Geometry: final body of the model. Coordinates: model frame, mm. A direction names the side the tool comes from. Coordinates: 2 decimals unless noted, no trailing zeros. Loops run counter-clockwise (first coordinate to the right, second up) from the corner with the lowest first, then second, coordinate; pieces in that order, holes last. Notation, with made-up numbers: (28, 6) -> (55, 6) arc R18 cw to (55, 11) -> close; hole circle Ø6 at (55, 34). An arc over 180 degrees is marked (long way). One line per item, written item: value. Start each with the question number.
Item 1: Section query B-B on y = 19. Return loops of the section in (x, z), then the cut area to 3 significant figures.
Item 2: Contact query for flat-ended pins moving along their axis: pin 1 Ø1 at (x, z) = (25, 22.5) entering from +Y; pin 2 Ø1.5 at (x, z) = (34.5, 24) entering from -Y; pin 3 Ø5 at (x, y) = (36.5, 11.5) entering from +Z; pin 4 Ø1.4 at (x, z) = (31.5, 23.5) entering from -Y. Output: stop coordinate, or through.
Item 3: Set-up query: faces 1 (the cylindrical face through (26.67, 8.68, 18.86)), 2 (the flat face through (32, 29.25, 21)), 3 (the flat face through (25, 29.25, 21)). Return all of +Z, -Z, +X, -X, +Y, -Y with unobstructed straight access to the full face (end or side cutting, diameter ignored); none if empty.
Item 4: Section query C-C on z = 9.75. Give the number of separate pieces and of enclosed holes in the cut face, then the cut area to 3 significant figures.
Item 5: Section query A-A on x = 35. Return loops of the section in (y, z).
Item 6: Mould query, pull axis X, two halves, no side actions, for faces 4 (the flat face through (29, 35.5, 25)), 5 (the cylindrical face through (33.017, 38.57, 1.972)), 6 (the flat face through (25.915, 15, 14)), 7 (the flat face through (38.615, 21, 2)). Classes: +X half, -X half, draft (parallel to the pull), parting line (faces both ways), or undercut.
Item 7: Ray query, probe 1 along Y at (x, z) = (26.25, 14.75); probe 2 along Y at (x, z) = (28.5, 11); probe 3 along Y at (x, z) = (29.5, 25). Return the intervals inside material, ascending. Write a range as from..to.
from build123d import *

# Parameters (mm, degrees)
ESQUISSE1_W                                        = 14
ESQUISSE1_H                                        = 42.5
ESQUISSE1_R                                        = 1.6
BOSS_EXTRU_1_DEPTH                                 = 4
ESQUISSE2_W                                        = 8
ESQUISSE2_H                                        = 42.5
BOSS_EXTRU_2_DEPTH                                 = 24
ENL_V_MAT_EXTRU_1_DEPTH                            = 9
ENL_V_START                                        = -1.7
ENL_V_MAT_EXTRU_3_DEPTH                            = 1.7
ENL_V_START_2                                      = -1.3
ENL_V_MAT_EXTRU_4_DEPTH                            = 1.3
ESQUISSE6_W                                        = 12
ESQUISSE6_H                                        = 7
ENL_V_MAT_EXTRU_2_DEPTH                            = 9
CHAMBRAGE_POUR_VIS_T_TE_HEXAGONALE_M31_D           = 3.4
CHAMBRAGE_POUR_VIS_T_TE_HEXAGONALE_M31_DEPTH       = 30
CHAMBRAGE_POUR_VIS_T_TE_HEXAGONALE_M31_CBORE_D     = 6.5
CHAMBRAGE_POUR_VIS_T_TE_HEXAGONALE_M31_CBORE_DEPTH = 3.4
CHAMBRAGE_POUR_VIS_T_TE_HEXAGONALE_M31_TIP         = 1.021463052
TROU_POUR_TARAUDAGE_POUR_TROU_TARAUD_M3_D          = 2.5
TROU_POUR_TARAUDAGE_POUR_TROU_TARAUD_M3_DEPTH      = 34.5
ENL_V_MAT_EXTRU_5_DEPTH                            = 4.1
ENL_V_MAT_EXTRU_6_DEPTH                            = 24
TROU_POUR_TARAUDAGE_POUR_TROU_TARAUD_2_D           = 2.5
TROU_POUR_TARAUDAGE_POUR_TROU_TARAUD_2_DEPTH       = 5


with BuildPart() as part:
    # Esquisse1 → Boss.-Extru.1 (new body)
    with BuildSketch(Plane.XY):
        with Locations((31.615489842, 21.249999998)):
            Rectangle(ESQUISSE1_W, ESQUISSE1_H)
        with Locations((34.615489842, 3.999999998)):
            Circle(ESQUISSE1_R, mode=Mode.SUBTRACT)
        with Locations((34.615489842, 38.499999998)):
            Circle(ESQUISSE1_R, mode=Mode.SUBTRACT)
    extrude(amount=BOSS_EXTRU_1_DEPTH)

    # Esquisse2 → Boss.-Extru.2 (add)
    with BuildSketch(Plane.XY.offset(4)):
        with Locations((28.615489842, 21.249999998)):
            Rectangle(ESQUISSE2_W, ESQUISSE2_H)
    extrude(amount=BOSS_EXTRU_2_DEPTH)

    # Esquisse3 → Enlèv. mat.-Extru.1 (cut, through all)
    with BuildSketch(Plane(origin=(32.615489842, 0, 0), x_dir=(0, 0, -1), z_dir=(1, 0, 0))):
        with BuildLine():
            Line((-13, 27.250000778), (-28, 27.250000778))
            Line((-28, 27.250000778), (-28, 15.250000778))
            Line((-28, 15.250000778), (-13, 15.250000778))
            ThreePointArc((-13, 15.250000778), (-7, 21.250000778), (-13, 27.250000778))
        make_face()
    extrude(amount=-ENL_V_MAT_EXTRU_1_DEPTH, mode=Mode.SUBTRACT)

    # Esquisse7 → Enlèv. mat.-Extru.3 (cut)
    with BuildSketch(Plane(origin=(32.615489842, 0, 0), x_dir=(0, 0, -1), z_dir=(1, 0, 0)).offset(ENL_V_START)):
        with BuildLine():
            Line((-13, 13.250000429), (-28, 13.250000429))
            Line((-28, 13.250000429), (-28, 29.250000429))
            Line((-28, 29.250000429), (-13, 29.250000429))
            ThreePointArc((-13, 29.250000429), (-5, 21.250000429), (-13, 13.250000429))
        make_face()
    extrude(amount=ENL_V_MAT_EXTRU_3_DEPTH, mode=Mode.SUBTRACT)

    # Esquisse8 → Enlèv. mat.-Extru.4 (cut)
    with BuildSketch(Plane.ZY.offset(-24.615489842).offset(ENL_V_START_2)):
        with BuildLine():
            Line((13, 13.250000429), (28, 13.250000429))
            Line((28, 13.250000429), (28, 29.250000429))
            Line((28, 29.250000429), (13, 29.250000429))
            ThreePointArc((13, 29.250000429), (5, 21.250000429), (13, 13.250000429))
        make_face()
    extrude(amount=ENL_V_MAT_EXTRU_4_DEPTH, mode=Mode.SUBTRACT)

    # Esquisse6 → Enlèv. mat.-Extru.2 (cut, through all)
    with BuildSketch(Plane(origin=(32.615489842, 0, 0), x_dir=(0, 0, -1), z_dir=(1, 0, 0))):
        with Locations((-22, 38.999999998)):
            Rectangle(ESQUISSE6_W, ESQUISSE6_H)
        Polygon((-28, -2e-09), (-16, 0), (-16, 7), (-28, 7), align=None)
    extrude(amount=-ENL_V_MAT_EXTRU_2_DEPTH, mode=Mode.SUBTRACT)

    # Chambrage pour vis à tête hexagonale M31
    with Locations(Plane(origin=(0, 7, 0), x_dir=(-1, 0, 0), z_dir=(0, -1, 0))):
        with Locations((-28.415489842, -21.6)):
            CounterBoreHole(CHAMBRAGE_POUR_VIS_T_TE_HEXAGONALE_M31_D / 2, CHAMBRAGE_POUR_VIS_T_TE_HEXAGONALE_M31_CBORE_D / 2, CHAMBRAGE_POUR_VIS_T_TE_HEXAGONALE_M31_CBORE_DEPTH, depth=CHAMBRAGE_POUR_VIS_T_TE_HEXAGONALE_M31_DEPTH)
            with Locations((0, 0, -(CHAMBRAGE_POUR_VIS_T_TE_HEXAGONALE_M31_DEPTH + CHAMBRAGE_POUR_VIS_T_TE_HEXAGONALE_M31_TIP / 2))):  # 118° drill point
                Cone(0, CHAMBRAGE_POUR_VIS_T_TE_HEXAGONALE_M31_D / 2, CHAMBRAGE_POUR_VIS_T_TE_HEXAGONALE_M31_TIP, mode=Mode.SUBTRACT)

    # Trou pour taraudage pour trou taraud_ M3
    with Locations(Plane.XY.offset(16)):
        with Locations((28.615489842, 4), (28.615489842, 38.499999998)):
            Hole(TROU_POUR_TARAUDAGE_POUR_TROU_TARAUD_M3_D / 2, depth=TROU_POUR_TARAUDAGE_POUR_TROU_TARAUD_M3_DEPTH)

    # Esquisse15 → Enlèv. mat.-Extru.5 (cut)
    with BuildSketch(Plane(origin=(0, 35.499999998, 0), x_dir=(1, 0, 0), z_dir=(0, 1, 0))):
        Polygon((25.297858374, -21.619339993), (26.873423034, -24.309618047), (29.991054501, -24.290278053), (31.533121309, -21.580660007), (29.95755665, -18.890381953), (26.839925183, -18.909721947), align=None)
    extrude(amount=-ENL_V_MAT_EXTRU_5_DEPTH, mode=Mode.SUBTRACT)

    # Esquisse16 → Enlèv. mat.-Extru.6 (cut)
    with BuildSketch(Plane.XY.offset(28)):
        with BuildLine():
            Line((30.615489842, 0), (32.615489842, -2e-09))
            Line((32.615489842, -2e-09), (32.615489842, 13.250000429))
            add(Edge.make_bspline(
                [(32.615489842, 13.250000429), (32.591528482, 1.687598594), (30.638844219, 5.520365059), (30.615489842, 0)],
                knots=[0, 0, 0, 0, 1, 1, 1, 1], degree=3))
        make_face()
        with BuildLine():
            Line((30.615489842, 42.500000857), (32.615489842, 42.50000086))
            Line((32.615489842, 42.50000086), (32.615489842, 29.250000429))
            add(Edge.make_bspline(
                [(32.615489842, 29.250000429), (32.591528482, 40.812402263), (30.638844219, 36.979635798), (30.615489842, 42.500000857)],
                knots=[0, 0, 0, 0, 1, 1, 1, 1], degree=3))
        make_face()
    extrude(amount=-ENL_V_MAT_EXTRU_6_DEPTH, mode=Mode.SUBTRACT)

    # Trou pour taraudage pour trou taraud 2
    with Locations(Plane.XY.offset(28)):
        with Locations((28.450357355, 33.249999999), (28.450357355, 9.249999999)):
            Hole(TROU_POUR_TARAUDAGE_POUR_TROU_TARAUD_2_D / 2, depth=TROU_POUR_TARAUDAGE_POUR_TROU_TARAUD_2_DEPTH)


solid = part.part
Reply:
1. outline: (24.62, 0) -> (38.62, 0) -> (38.62, 4) -> (32.62, 4) -> (32.62, 5.32) -> (30.92, 5.32) -> (30.92, 7.44) -> (25.92, 7.44) -> (25.92, 5.32) -> (24.62, 5.32) -> close
1. area: 77.2 mm²
2. pin 1: stops at y = 35.5
2. pin 2: passes through
2. pin 3: stops at z = 4
2. pin 4: stops at y = 7
3. face 1: -Y
3. face 2: +Z, +X
3. face 3: +Z, -X
4. separate pieces: 2
4. enclosed holes: 2
4. area: 217 mm²
5. outline: (0, 0) -> (2.45, 0) -> (2.45, 4) -> (0, 4) -> close; (5.55, 0) -> (36.95, 0) -> (36.95, 4) -> (5.55, 4) -> close; (40.05, 0) -> (42.5, 0) -> (42.5, 4) -> (40.05, 4) -> close
6. face 4: draft
6. face 5: undercut
6. face 6: -X half
6. face 7: +X half
7. probe 1: y = 0..15.25, 27.25..42.5
7. probe 2: y = 0..2.76, 5.24..15.59, 26.91..37.26, 39.74..42.5
7. probe 3: y = 7..8.57, 9.93..15.25, 27.25..32.57, 33.93..35.5
